Check sheet for the modelled part. Datum: model origin and axes. Units: mm. Face numbers are marked on the shaded views. A direction names the side the tool comes from. Give positions to 0.01 mm unless a question says otherwise; leave off trailing zeros. Write each loop counter-clockwise with the first axis right and the second up, starting at its lowest first coordinate (ties: lowest second). Pieces come first, ordered by that corner, then holes. Notation, with made-up numbers: (-29, -32.75) -> (-2, -32.75) arc R34 ccw to (-2, 3.25) -> close; hole circle Ø6 at (5, -27.5). An arc over 180 degrees is marked (long way). Return JSON: item names as keys, results as strings.
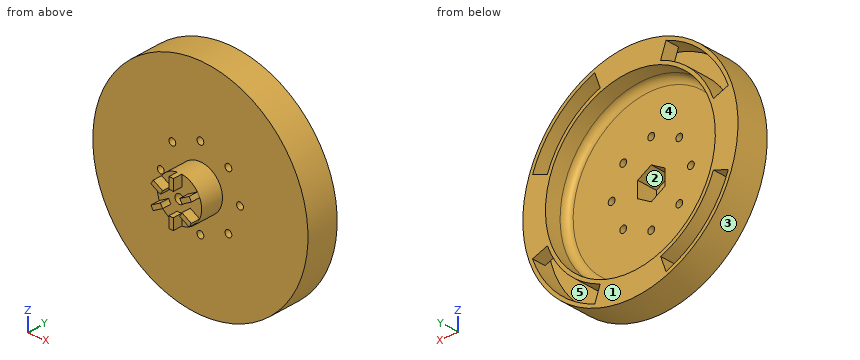
from build123d import *

# Parameters (mm, degrees)
SKETCH_1_R               = 21.5
SKETCH_1_R_2             = 1.5
EXTRUDE_1_DEPTH          = 4
SKETCH_9_R               = 9.75
EXTRUDE_4_DEPTH          = 5
SKETCH_10_R              = 9.75
SKETCH_10_R_2            = 2
EXTRUDE_5_DEPTH          = 5
EXTRUDE_6_DEPTH          = 4
PATTERN_CIRCULAR_1_COUNT = 2
PATTERN_CIRCULAR_1_ANGLE = 60
EXTRUDE_START            = -4
SKETCH_12_R              = 47.5
SKETCH_12_R_2            = 21.5
EXTRUDE_7_DEPTH          = 4
SKETCH_13_R              = 47.5
SKETCH_13_R_2            = 46
SKETCH_13_R_3            = 39
SKETCH_13_R_4            = 37.5
EXTRUDE_8_DEPTH          = 10
EXTRUDE_START_2          = -6
EXTRUDE_9_DEPTH          = 6
FILLET_1_R               = 3


with BuildPart() as part:
    # 草图1 → 凸台-拉伸1 (new body)
    with BuildSketch(Plane(origin=(0, 0, 0), x_dir=(1, 0, 0), z_dir=(0, 1, 0))):
        with Locations(Location((0, 0, 0), (0, 0, 270))):
            Circle(SKETCH_1_R)
        with Locations(Location((12.374368671, 12.374368671, 0), (0, 0, 270))):
            Circle(SKETCH_1_R_2, mode=Mode.SUBTRACT)
        with Locations(Location((12.374368671, -12.374368671, 0), (0, 0, 90))):
            Circle(SKETCH_1_R_2, mode=Mode.SUBTRACT)
        with Locations(Location((-12.374368671, -12.374368671, 0), (0, 0, 270))):
            Circle(SKETCH_1_R_2, mode=Mode.SUBTRACT)
        with Locations(Location((-12.374368671, 12.374368671, 0), (0, 0, 90))):
            Circle(SKETCH_1_R_2, mode=Mode.SUBTRACT)
        with Locations(Location((0, 17.5, 0), (0, 0, 90))):
            Circle(SKETCH_1_R_2, mode=Mode.SUBTRACT)
        with Locations(Location((17.5, 0, 0), (0, 0, 270))):
            Circle(SKETCH_1_R_2, mode=Mode.SUBTRACT)
        with Locations(Location((0, -17.5, 0), (0, 0, 90))):
            Circle(SKETCH_1_R_2, mode=Mode.SUBTRACT)
        with Locations(Location((-17.5, 0, 0), (0, 0, 270))):
            Circle(SKETCH_1_R_2, mode=Mode.SUBTRACT)
        Polygon((0, 6.899335717), (-5.975, 3.449667858), (-5.975, -3.449667858), (0, -6.899335717), (5.975, -3.449667858), (5.975, 3.449667858), align=None, mode=Mode.SUBTRACT)
    extrude(amount=EXTRUDE_1_DEPTH)

    # 草图9 → 凸台-拉伸4 (add)
    with BuildSketch(Plane.XZ):
        with Locations(Location((0, 0, 0), (0, 0, 270))):
            Circle(SKETCH_9_R)
        Polygon((-5.975, -3.449667858), (-5.975, 3.449667858), (0, 6.899335717), (5.975, 3.449667858), (5.975, -3.449667858), (0, -6.899335717), align=None, mode=Mode.SUBTRACT)
    extrude(amount=EXTRUDE_4_DEPTH)

    # 草图10 → 凸台-拉伸5 (add)
    with BuildSketch(Plane.XZ.offset(5)):
        with Locations(Location((0, 0, 0), (0, 0, 270))):
            Circle(SKETCH_10_R)
        with Locations(Location((0, 0, 0), (0, 0, 270))):
            Circle(SKETCH_10_R_2, mode=Mode.SUBTRACT)
    extrude(amount=EXTRUDE_5_DEPTH)

    # 草图11 → 凸台-拉伸6 (add)
    with BuildSketch(Plane.XZ.offset(10)):
        with BuildLine():
            Line((-7.899218714, -5.715316589), (-3.742640687, -3.315515147))
            ThreePointArc((-3.742640687, -3.315515147), (-4.330127019, -2.5), (-4.742640687, -1.583464339))
            Line((-4.742640687, -1.583464339), (-8.899218714, -3.983265782))
            ThreePointArc((-8.899218714, -3.983265782), (-8.443747687, -4.875), (-7.899218714, -5.715316589))
        make_face()
        with BuildLine():
            ThreePointArc((-1, 4.898979486), (0, 5), (1, 4.898979486))
            Line((1, 4.898979486), (1, 9.698582371))
            ThreePointArc((1, 9.698582371), (0, 9.75), (-1, 9.698582371))
            Line((-1, 9.698582371), (-1, 4.898979486))
        make_face()
        with BuildLine():
            Line((8.899218714, -3.983265782), (4.742640687, -1.583464339))
            ThreePointArc((4.742640687, -1.583464339), (4.330127019, -2.5), (3.742640687, -3.315515147))
            Line((3.742640687, -3.315515147), (7.899218714, -5.715316589))
            ThreePointArc((7.899218714, -5.715316589), (8.443747687, -4.875), (8.899218714, -3.983265782))
        make_face()
    extrude_6 = extrude(amount=EXTRUDE_6_DEPTH)

    # 阵列(圆周)1: 凸台-拉伸6 ×2 about axis
    pattern_circular_1_axis = Axis((0, 0, 0), (0, -1, 0))
    for i in range(1, PATTERN_CIRCULAR_1_COUNT):
        add(extrude_6.rotate(pattern_circular_1_axis, i * PATTERN_CIRCULAR_1_ANGLE / (PATTERN_CIRCULAR_1_COUNT - 1)))

    # 草图12 → 凸台-拉伸7 (add)
    with BuildSketch(Plane(origin=(0, 4, 0), x_dir=(1, 0, 0), z_dir=(0, 1, 0)).offset(EXTRUDE_START)):
        with Locations(Location((0, 0, 0), (0, 0, 270))):
            Circle(SKETCH_12_R)
        Circle(SKETCH_12_R_2, mode=Mode.SUBTRACT)
    extrude(amount=EXTRUDE_7_DEPTH)

    # 草图13 → 凸台-拉伸8 (add)
    # profile 1 of 2: a face of its own
    with BuildSketch(Plane(origin=(0, 4, 0), x_dir=(1, 0, 0), z_dir=(0, 1, 0))):
        with Locations(Location((0, 0, 0), (0, 0, 270))):
            Circle(SKETCH_13_R)
        with Locations(Location((0, 0, 0), (0, 0, 270))):
            Circle(SKETCH_13_R_2, mode=Mode.SUBTRACT)
    # profile 2 of 2: a face of its own
    with BuildSketch(Plane(origin=(0, 4, 0), x_dir=(1, 0, 0), z_dir=(0, 1, 0))):
        with Locations(Location((0, 0, 0), (0, 0, 270))):
            Circle(SKETCH_13_R_3)
        with Locations(Location((0, 0, 0), (0, 0, 270))):
            Circle(SKETCH_13_R_4, mode=Mode.SUBTRACT)
    extrude(amount=EXTRUDE_8_DEPTH)

    # 草图14 → 凸台-拉伸9 (add)
    with BuildSketch(Plane(origin=(0, 14, 0), x_dir=(1, 0, 0), z_dir=(0, 1, 0)).offset(EXTRUDE_START_2)):
        with BuildLine():
            Line((-15.732926593, 43.225860556), (-13.33878559, 36.648012211))
            ThreePointArc((-13.33878559, 36.648012211), (0, 39), (13.33878559, 36.648012211))
            Line((13.33878559, 36.648012211), (15.732926593, 43.225860556))
            ThreePointArc((15.732926593, 43.225860556), (0, 46), (-15.732926593, 43.225860556))
        make_face()
        with BuildLine():
            Line((43.225860556, -15.732926593), (36.648012211, -13.33878559))
            ThreePointArc((36.648012211, -13.33878559), (39, 0), (36.648012211, 13.33878559))
            Line((36.648012211, 13.33878559), (43.225860556, 15.732926593))
            ThreePointArc((43.225860556, 15.732926593), (46, 0), (43.225860556, -15.732926593))
        make_face()
        with BuildLine():
            Line((-15.732926593, -43.225860556), (-13.33878559, -36.648012211))
            ThreePointArc((-13.33878559, -36.648012211), (0, -39), (13.33878559, -36.648012211))
            Line((13.33878559, -36.648012211), (15.732926593, -43.225860556))
            ThreePointArc((15.732926593, -43.225860556), (0, -46), (-15.732926593, -43.225860556))
        make_face()
        with BuildLine():
            Line((-43.225860556, 15.732926593), (-36.648012211, 13.33878559))
            ThreePointArc((-36.648012211, 13.33878559), (-39, 0), (-36.648012211, -13.33878559))
            Line((-36.648012211, -13.33878559), (-43.225860556, -15.732926593))
            ThreePointArc((-43.225860556, -15.732926593), (-46, 0), (-43.225860556, 15.732926593))
        make_face()
    extrude(amount=EXTRUDE_9_DEPTH)

    # 圆角1
    fillet_1_edges = [part.edges().sort_by_distance(p)[0] for p in [
        (0, 4, -37.5),
    ]]
    fillet(fillet_1_edges, radius=FILLET_1_R)


solid = part.part
(1) Cross-section at C-C on x = -41.5. Enter the section's corners in (y, z), then the cut area to 3 significant figures.
Reply:
{"outline": "(0, -23.11) -> (14, -23.11) -> (14, -19.84) -> (4, -19.84) -> (4, 19.84) -> (14, 19.84) -> (14, 23.11) -> (0, 23.11) -> close; (8, -15.1) -> (14, -15.1) -> (14, 15.1) -> (8, 15.1) -> close", "area": "431 mm^2"}
(2) Depth check by flat-ended pin: pin 1 Ø1.8 at (x, z) = (-17.5, 0) entering from -Y; pin 2 Ø4 at (y, z) = (-1.5, -14) entering from -X; pin 3 Ø3.5 at (x, z) = (-12.37, 12.37) entering from -Y; pin 4 Ø3.5 at (x, z) = (-2.5, -2.5) entering from +Y. Enter the tip coordinate at first touch or a pass-through.
Reply:
{"pin 1": "through", "pin 2": "x = -45.78", "pin 3": "y = 0", "pin 4": "y = -5"}
(3) Release check for a two-part mould opening along Y. For the marked faces 3, 4 and 5 record: pulls with the +Y half, pulls with the -Y half, needs draft (parallel to the pull), parting line crosses it, or undercut.
Reply:
{"face 3": "needs draft", "face 4": "pulls with the +Y half", "face 5": "undercut"}
(4) Cross-section at D-D on z = -8. State how many separate pieces and enclosed holes the cut face has, then the cut area to 3 significant figures.
Reply:
{"separate pieces": "1", "enclosed holes": "2", "area": "645 mm^2"}
(5) Set-up check for the marked faces 1 and 2: record each of +Z, -Z, +X, -X, +Y, -Y from which the full face is reachable in a straight line by a thin tool's end or side.
Reply:
{"face 1": "+Z, -Z, +X, -X, +Y", "face 2": "+Y"}
(6) Cross-section at A-A on y = 12. Enter the section's corners in (x, z), then the cut area to 3 significant figures.
Reply:
{"outline": "circle Ø95 at (0, 0); hole (-43.23, -15.73) arc R46 ccw to (-15.73, -43.23) -> (-13.34, -36.65) arc R39 cw to (-36.65, -13.34) -> close; hole (-43.23, 15.73) -> (-36.65, 13.34) arc R39 cw to (-13.34, 36.65) -> (-15.73, 43.23) arc R46 ccw to start; hole circle Ø75 at (0, 0); hole (13.34, -36.65) -> (15.73, -43.23) arc R46 ccw to (43.23, -15.73) -> (36.65, -13.34) arc R39 cw to start; hole (13.34, 36.65) arc R39 cw to (36.65, 13.34) -> (43.23, 15.73) arc R46 ccw to (15.73, 43.23) -> close", "area": "1,630 mm^2"}
(7) Cross-section at B-B on y = -1.5. Enter the section's corners in (x, z) (3 decimals).
Reply:
{"outline": "circle Ø19.5 at (0, 0); hole (-5.975, -3.45) -> (0, -6.899) -> (5.975, -3.45) -> (5.975, 3.45) -> (0, 6.899) -> (-5.975, 3.45) -> close"}
(8) Thickness scan on L1, parallel to X at y = 7.25, z = 0; L2, parallel to X at y = 3.1, z = 0 (3 decimals); L3, parallel to Z at x = 30.5, y = 5. Record the ranges inside material, lowest first.
Reply:
{"L1": "-47.5 to -46, -39 to -37.5, 37.5 to 39, 46 to 47.5", "L2": "-47.5 to -19, -16 to -5.975, 5.975 to 16, 19 to 47.5", "L3": "-36.41 to -34.43, -24.31 to -20.48, 20.48 to 24.31, 34.43 to 36.41"}
